Read the model definition and answer for the solid it produces. Units are mm, in the model's axes. Round coordinates to 2 decimals unless told otherwise and drop trailing zeros. Order: outer loops, then holes, each group sorted by start corner. A loop starts at its lowest first (then second) coordinate and runs counter-clockwise, first axis right, second up.
from build123d import *

# Parameters (mm, degrees)
F0_R     = 1
F1_DEPTH = 2
F3_DEPTH = 2
F5_DEPTH = 60
F6_W     = 84.123355
F6_H     = 40.454367
F7_DEPTH = 4


with BuildPart() as f1:
    # F0 (on Top) → F1 (new body)
    with BuildSketch(Plane.XY):
        with BuildLine():
            Line((-3.751696, 3.78006), (-3.109909, 2.896716))
            ThreePointArc((-3.109909, 2.896716), (-3.438322, 2.498087), (-3.715956, 2.062565))
            Line((-3.715956, 2.062565), (-4.754388, 2.399972))
            Line((-4.754388, 2.399972), (-5.817595, 2.320708))
            Line((-5.817595, 2.320708), (-6.070611, 1.542005))
            Line((-6.070611, 1.542005), (-5.257049, 0.852941))
            Line((-5.257049, 0.852941), (-4.218616, 0.515534))
            ThreePointArc((-4.218616, 0.515534), (-4.25, 0), (-4.218616, -0.515534))
            Line((-4.218616, -0.515534), (-5.257049, -0.852941))
            Line((-5.257049, -0.852941), (-6.070611, -1.542005))
            Line((-6.070611, -1.542005), (-5.817595, -2.320708))
            Line((-5.817595, -2.320708), (-4.754388, -2.399972))
            Line((-4.754388, -2.399972), (-3.715956, -2.062565))
            ThreePointArc((-3.715956, -2.062565), (-3.438322, -2.498087), (-3.109909, -2.896716))
            Line((-3.109909, -2.896716), (-3.751696, -3.78006))
            Line((-3.751696, -3.78006), (-4.00486, -4.815724))
            Line((-4.00486, -4.815724), (-3.342456, -5.296989))
            Line((-3.342456, -5.296989), (-2.435713, -4.736177))
            Line((-2.435713, -4.736177), (-1.793926, -3.852834))
            ThreePointArc((-1.793926, -3.852834), (-1.313322, -4.04199), (-0.813322, -4.171451))
            Line((-0.813322, -4.171451), (-0.813322, -5.263324))
            Line((-0.813322, -5.263324), (-0.409388, -6.25))
            Line((-0.409388, -6.25), (0.409388, -6.25))
            Line((0.409388, -6.25), (0.813322, -5.263324))
            Line((0.813322, -5.263324), (0.813322, -4.171451))
            ThreePointArc((0.813322, -4.171451), (1.313322, -4.04199), (1.793926, -3.852834))
            Line((1.793926, -3.852834), (2.435713, -4.736177))
            Line((2.435713, -4.736177), (3.342456, -5.296989))
            Line((3.342456, -5.296989), (4.00486, -4.815724))
            Line((4.00486, -4.815724), (3.751696, -3.78006))
            Line((3.751696, -3.78006), (3.109909, -2.896716))
            ThreePointArc((3.109909, -2.896716), (3.438322, -2.498087), (3.715956, -2.062565))
            Line((3.715956, -2.062565), (4.754388, -2.399972))
            Line((4.754388, -2.399972), (5.817595, -2.320708))
            Line((5.817595, -2.320708), (6.070611, -1.542005))
            Line((6.070611, -1.542005), (5.257049, -0.852941))
            Line((5.257049, -0.852941), (4.218616, -0.515534))
            ThreePointArc((4.218616, -0.515534), (4.25, 0), (4.218616, 0.515534))
            Line((4.218616, 0.515534), (5.257049, 0.852941))
            Line((5.257049, 0.852941), (6.070611, 1.542005))
            Line((6.070611, 1.542005), (5.817595, 2.320708))
            Line((5.817595, 2.320708), (4.754388, 2.399972))
            Line((4.754388, 2.399972), (3.715956, 2.062565))
            ThreePointArc((3.715956, 2.062565), (3.438322, 2.498087), (3.109909, 2.896716))
            Line((3.109909, 2.896716), (3.751696, 3.78006))
            Line((3.751696, 3.78006), (4.00486, 4.815724))
            Line((4.00486, 4.815724), (3.342456, 5.296989))
            Line((3.342456, 5.296989), (2.435713, 4.736177))
            Line((2.435713, 4.736177), (1.793926, 3.852834))
            ThreePointArc((1.793926, 3.852834), (1.313322, 4.04199), (0.813322, 4.171451))
            Line((0.813322, 4.171451), (0.813322, 5.263324))
            Line((0.813322, 5.263324), (0.409388, 6.25))
            Line((0.409388, 6.25), (-0.409388, 6.25))
            Line((-0.409388, 6.25), (-0.813322, 5.263324))
            Line((-0.813322, 5.263324), (-0.813322, 4.171451))
            ThreePointArc((-0.813322, 4.171451), (-1.313322, 4.04199), (-1.793926, 3.852834))
            Line((-1.793926, 3.852834), (-2.435713, 4.736177))
            Line((-2.435713, 4.736177), (-3.342456, 5.296989))
            Line((-3.342456, 5.296989), (-4.00486, 4.815724))
            Line((-4.00486, 4.815724), (-3.751696, 3.78006))
        make_face()
        Circle(F0_R, mode=Mode.SUBTRACT)
    extrude(amount=F1_DEPTH)

    # F2 (on face) → F3 (join)
    with BuildSketch(Plane.XY.offset(2)):
        with BuildLine():
            ThreePointArc((-34.301606, -7.25), (-24.988946, 4.275), (-15.676287, -7.25))
            Line((-15.676287, -7.25), (-14.172292, -7.25))
            ThreePointArc((-14.172292, -7.25), (-14.124852, -3.526211), (-15.322639, 0))
            Line((-15.322639, 0), (-5.88111, 2.12523))
            Line((-5.88111, 2.12523), (-5.817595, 2.320708))
            Line((-5.817595, 2.320708), (-4.754388, 2.399972))
            Line((-4.754388, 2.399972), (-4.715983, 2.387493))
            Line((-4.715983, 2.387493), (-3.27176, 2.712579))
            ThreePointArc((-3.27176, 2.712579), (-3.192163, 2.805815), (-3.109909, 2.896716))
            Line((-3.109909, 2.896716), (-3.751696, 3.78006))
            Line((-3.751696, 3.78006), (-4.00486, 4.815724))
            Line((-4.00486, 4.815724), (-3.342456, 5.296989))
            Line((-3.342456, 5.296989), (-2.435713, 4.736177))
            Line((-2.435713, 4.736177), (-1.793926, 3.852834))
            ThreePointArc((-1.793926, 3.852834), (-1.313322, 4.04199), (-0.813322, 4.171451))
            Line((-0.813322, 4.171451), (-0.813322, 5.263324))
            Line((-0.813322, 5.263324), (-0.453438, 6.142401))
            Line((-0.453438, 6.142401), (-18.813315, 3.852834))
            ThreePointArc((-18.813315, 3.852834), (-31.005839, 3.958528), (-35.8056, -7.25))
            Line((-35.8056, -7.25), (-34.301606, -7.25))
        make_face()
    extrude(amount=-F3_DEPTH)

    # F4 (on face) → F5 (join)
    with BuildSketch(Plane.XY.offset(2)):
        with BuildLine():
            Line((-15.676287, -7.25), (-14.172292, -7.25))
            ThreePointArc((-14.172292, -7.25), (-14.124852, -3.526211), (-15.322639, 0))
            ThreePointArc((-15.322639, 0), (-16.837085, 2.135605), (-18.813315, 3.852834))
            ThreePointArc((-18.813315, 3.852834), (-31.005839, 3.958528), (-35.8056, -7.25))
            Line((-35.8056, -7.25), (-34.301606, -7.25))
            ThreePointArc((-34.301606, -7.25), (-24.988946, 4.275), (-15.676287, -7.25))
        make_face()
    extrude(amount=F5_DEPTH)

    # F6 (on Top) → F7 (cut)
    with BuildSketch(Plane.XY):
        with Locations((-13.661468, 5.350011)):
            Rectangle(F6_W, F6_H)
    extrude(amount=F7_DEPTH, mode=Mode.SUBTRACT)


solid = f1.part
Q1. A cutting plane is placed at B-B, the plane z = 29. Give the vertices of the cut face in (x, y) (3 decimals).
Outcome:
outline: (-35.806, -7.25) - (-34.302, -7.25) arc R9.525 cw (long way) to (-15.676, -7.25) - (-14.172, -7.25) arc R11 ccw to (-15.323, 0) arc R11 ccw to (-18.813, 3.853) arc R11 ccw to start
Q2. Straight lines are drawn through the part: probe 1 along X at (y, z) = (-5.25, 36.5); probe 2 along X at (y, z) = (3.5, 52.5); probe 3 along Y at (x, z) = (-20.25, 35.5). For each, find the intervals that lie inside material, in ascending order.
Outcome:
probe 1: x = -35.99 to -34.51, -15.46 to -13.99
probe 2: x = -31.66 to -28.75, -21.23 to -18.32
probe 3: y = 3.01 to 4.68
Q3. For a pull along Y with two mould halves and no side action, classify faces 1 (the face through (-25.23, 4.27, 32.59)), 2 (the face through (-15, -7.25, 33)), 3 (the face through (-25, 5, 62)) as released by +Y, released by -Y, zero draft, split by the parting line, or undercut.
Outcome:
face 1: undercut
face 2: released by -Y
face 3: zero draft
Q4. A cutting plane is placed at C-C, the plane y = -2.75. Give the vertices of the cut face in (x, z), plus the area to 3 significant figures.
Outcome:
outline: (-35.7, 4) - (-34.18, 4) - (-34.18, 62) - (-35.7, 62) - close; (-15.8, 4) - (-14.28, 4) - (-14.28, 62) - (-15.8, 62) - close
area: 176 mm2
Q5. A cutting plane is placed at A-A, the plane y = -5.25. Give the vertices of the cut face in (x, z).
Outcome:
outline: (-35.99, 4) - (-34.51, 4) - (-34.51, 62) - (-35.99, 62) - close; (-15.46, 4) - (-13.99, 4) - (-13.99, 62) - (-15.46, 62) - close
Q6. Flat-ended cylindrical pins translate along their axes: pin 1 (2 mm diameter, centred on y = 2.5, z = 34, fed in from +X); pin 2 (3 mm diameter, centred on x = -33, z = 48.5, fed in from +Y); pin 3 (4 mm diameter, centred on x = -28, z = 24.5, fed in from +Y). Find the tip coordinate at first contact, or state that the pin passes through.
Outcome:
pin 1: stops at x = -16.3
pin 2: stops at y = 3.62
pin 3: stops at y = 5.7
Q7. A cutting plane is placed at D-D, the plane x = -17.75. Give the vertices of the cut face in (y, z).
Outcome:
outline: (0.94, 4) - (3.03, 4) - (3.03, 62) - (0.94, 62) - close
